from build123d import *

# Parameters (mm, degrees)
F0_W     = 150
F0_H     = 350
F1_DEPTH = 5
F2_R     = 50
F3_DEPTH = 5
F2_R_2   = 55
F4_DEPTH = 20


with BuildPart() as f1:
    # F0 (on Top) → F1 (new body)
    with BuildSketch(Plane.XY):
        Rectangle(F0_W, F0_H)
    extrude(amount=F1_DEPTH)

    # F2 (on face) → F3 (cut, through all)
    with BuildSketch(Plane.XY.offset(5)):
        Circle(F2_R)
    extrude(amount=-F3_DEPTH, mode=Mode.SUBTRACT)

    # F2 (on face) → F4 (join)
    with BuildSketch(Plane.XY.offset(5)):
        Circle(F2_R_2)
        Circle(F2_R, mode=Mode.SUBTRACT)
    extrude(amount=F4_DEPTH)


solid = f1.part
Here's how the part is built. I have some questions about the finished solid (model axes, mm). Coordinates: 2 decimals unless noted, no trailing zeros. Loops run counter-clockwise (first coordinate to the right, second up) from the corner with the lowest first, then second, coordinate; pieces in that order, holes last. Notation, with made-up numbers: (29.25, 76.5) -> (33.25, 76.5) arc R20 cw to (33.25, 95.5) -> close; hole circle Ø1 at (-22, 65). An arc over 180 degrees is marked (long way). Use one line per item in the form item = value. Start each with the question number.
(1) If we section it at B-B (x = 38): Please give me the cut outline in (y, z).
(2) We'd pull the mould along X, two halves only. Please class faces 1 (the face through (-11.923, -53.692, 14.86)), 2 (the face through (47.69, 15.02, 12.32)), 3 (the face through (12, -49, 25)): pulls with the +X half, pulls with the -X half, needs draft (parallel to the pull), parting line crosses it, or undercut.
(3) Please list where these lines run through material, in increasing order: line 1 along Y through (x, z) = (0, 13.5); line 2 along Z through (x, y) = (9.5, 78.5); line 3 along X through (y, z) = (-10.5, 11).
(4) If we section it at A-A (y = 0): Please give me the cut outline in (x, z).
(5) If we section it at C-C (z = 13.75): Please give me the cut outline in (x, y).
(6) Will these pins go through, and if not, where does the flat tip stop? pin 1 (1 mm diameter, centred on x = 15.5, z = 22.5, fed in from -Y) (3 decimals); pin 2 (1 mm diameter, centred on x = 25, z = 20.5, fed in from +Y); pin 3 (12 mm diameter, centred on x = -17, z = 12, fed in from +Y).
(7) If we section it at D-D (y = 148.5): Please give me the cut outline in (x, z), then the cut area to 3 significant figures.
Verdict:
q1.outline = (-175, 0) -> (-32.5, 0) -> (-32.5, 25) -> (-39.76, 25) -> (-39.76, 5) -> (-175, 5) -> close; (32.5, 0) -> (175, 0) -> (175, 5) -> (39.76, 5) -> (39.76, 25) -> (32.5, 25) -> close
q2.face_1 = parting line crosses it
q2.face_2 = undercut
q2.face_3 = needs draft
q3.line_1 = -55 to -50, 50 to 55
q3.line_2 = 0 to 5
q3.line_3 = -53.99 to -48.89, 48.89 to 53.99
q4.outline = (-75, 0) -> (-50, 0) -> (-50, 25) -> (-55, 25) -> (-55, 5) -> (-75, 5) -> close; (50, 0) -> (75, 0) -> (75, 5) -> (55, 5) -> (55, 25) -> (50, 25) -> close
q5.outline = circle Ø110 at (0, 0); hole circle Ø100 at (0, 0)
q6.pin_1 = -52.915
q6.pin_2 = 49.24
q6.pin_3 = 53.89
q7.outline = (-75, 0) -> (75, 0) -> (75, 5) -> (-75, 5) -> close
q7.area = 750 mm²
